The model under review builds one solid part; all positions refer to its coordinate system, in mm. Face numbers are marked on the shaded views. A direction names the side the tool comes from. Give positions to 0.01 mm unless a question says otherwise; leave off trailing zeros. Loops run counter-clockwise (first coordinate to the right, second up) from the corner with the lowest first, then second, coordinate; pieces in that order, holes last. Notation, with made-up numbers: (45, 74.5) - (89, 74.5) arc R11 ccw to (89, 82.5) - close; hole circle Ø6 at (45, 53.5). An arc over 180 degrees is marked (long way). Return JSON: item names as keys, results as strings. Group by question number.
```python
from build123d import *

# Parameters (mm, degrees)
EXTRUDE_1_DEPTH            = 48
CUT_EXTRUDE_2_REACH        = 96.508
CUT_EXTRUDE_2_START_RADIUS = 70
CUT_EXTRUDE_2_END_RADIUS   = 70
SKETCH_3_W                 = 58.404028666
SKETCH_3_H                 = 6
EXTRUDE_2_DEPTH            = 13
CUT_EXTRUDE_3_DEPTH        = 140.034418617
CUT_EXTRUDE_3_DEPTH_BACK   = 140.034418617
SKETCH_4_W                 = 25
SKETCH_4_H                 = 38
SKETCH_4_W_2               = 40
SKETCH_4_H_2               = 25
CHAMFER_1_SIZE             = 5
CHAMFER_1_SIZE2            = 3.813196151
SKETCH_6_R                 = 6.5
CUT_EXTRUDE_4_DEPTH        = 2
SKETCH_7_R                 = 1.5
CUT_EXTRUDE_5_DEPTH        = 60
SKETCH_8_W                 = 9
SKETCH_8_H                 = 9
CUT_EXTRUDE_6_DEPTH        = 11
CUT_EXTRUDE_8_REACH        = 137.533
SKETCH_10_R                = 1
CUT_EXTRUDE_9_REACH        = 105.034
CUT_EXTRUDE_9_END_RADIUS   = 70
SKETCH_11_R                = 0.75
SKETCH_12_W                = 20
SKETCH_12_H                = 3
CUT_EXTRUDE_10_DEPTH       = 11
SKETCH_13_W                = 3.868283576
SKETCH_13_H                = 1.5
CUT_EXTRUDE_11_DEPTH       = 4
CUT_EXTRUDE_12_REACH       = 137.476


with BuildPart() as part:
    # 草图1 → 凸台-拉伸1 (new body)
    with BuildSketch(Plane(origin=(0, 0, 0), x_dir=(1, 0, 0), z_dir=(0, 1, 0))):
        with BuildLine():
            ThreePointArc((-9.396926208, -7.075874358), (-5.735764364, -11.847193368), (0, -13.655672925))
            Line((0, -13.655672925), (0, -5))
            ThreePointArc((0, -5), (-5, 0), (0, 5))
            Line((0, 5), (0, 70))
            ThreePointArc((0, 70), (-17.673593853, 67.732149533), (-34.202014333, 61.075545152))
            Line((-34.202014333, 61.075545152), (-9.396926208, -7.075874358))
        make_face()
        with BuildLine():
            Line((0, -5), (0, -13.655672925))
            ThreePointArc((0, -13.655672925), (5.735764364, -11.847193368), (9.396926208, -7.075874358))
            Line((9.396926208, -7.075874358), (34.202014333, 61.075545152))
            ThreePointArc((34.202014333, 61.075545152), (17.673593853, 67.732149533), (0, 70))
            Line((0, 70), (0, 5))
            ThreePointArc((0, 5), (3.535533906, 3.535533906), (5, 0))
            ThreePointArc((5, 0), (3.535533906, -3.535533906), (0, -5))
        make_face()
    extrude(amount=EXTRUDE_1_DEPTH)

    # 切除-拉伸2: from a cylinder face, 96.508 long prism both ways, kept between that surface and its translate by the depth
    cut_extrude_2_start = Plane(origin=(0, 5, 0), z_dir=(0, -1, 0)) * Cylinder(CUT_EXTRUDE_2_START_RADIUS, 334.016, mode=Mode.PRIVATE)
    cut_extrude_2_end = Plane(origin=(0, 5, 3), z_dir=(0, -1, 0)) * Cylinder(CUT_EXTRUDE_2_END_RADIUS, 334.016, mode=Mode.PRIVATE)
    # 草图3 → 切除-拉伸2 (cut, from a surface)
    with BuildSketch(Plane.XY, mode=Mode.PRIVATE) as cut_extrude_2_sk1:
        with Locations((3, 5)):
            Rectangle(SKETCH_3_W, SKETCH_3_H)
    cut_extrude_2_tool1 = extrude(cut_extrude_2_sk1.sketch, amount=CUT_EXTRUDE_2_REACH, both=True, mode=Mode.PRIVATE)
    add(((cut_extrude_2_tool1 & cut_extrude_2_start) - cut_extrude_2_end).solids().sort_by_distance((3, 5, -62.032204))[0], mode=Mode.SUBTRACT)

    # 草图2 → 凸台-拉伸2 (add)
    with BuildSketch(Plane(origin=(0, 48, 0), x_dir=(1, 0, 0), z_dir=(0, 1, 0))):
        Polygon((24.252642572, 33.739870901), (55.034455471, 118.312206771), (20.125623779, 80.877067961), (5.458790156, 40.580273767), align=None)
    extrude(amount=-EXTRUDE_2_DEPTH)

    # 草图4 → 切除-拉伸3 (cut, two sides: drawn at the far end of the back side and taken through both)
    with BuildSketch(Plane(origin=(0, 0, 0), x_dir=(0, 0, -1), z_dir=(1, 0, 0)).offset(-CUT_EXTRUDE_3_DEPTH_BACK)):
        with Locations((-1.155672925, 29)):
            Rectangle(SKETCH_4_W, SKETCH_4_H)
        with Locations((50.466884927, 22.5)):
            Rectangle(SKETCH_4_W_2, SKETCH_4_H_2)
    extrude(amount=CUT_EXTRUDE_3_DEPTH + CUT_EXTRUDE_3_DEPTH_BACK, mode=Mode.SUBTRACT)

    # 倒角1
    chamfer_1_edges = [part.edges().sort_by_distance(p)[0] for p in [
        (55.034455471, 41.5, -118.312206771),
    ]]
    chamfer_1_side = [part.faces().sort_by_distance(p)[0] for p in [
        (37.580039625, 41.5, -99.594637366),
    ]]
    chamfer(chamfer_1_edges, length=CHAMFER_1_SIZE, length2=CHAMFER_1_SIZE2, reference=chamfer_1_side[0])

    # 草图6 → 切除-拉伸4 (cut)
    with BuildSketch(Plane.XZ):
        with Locations(Location((0, 0, 0), (0, 0, 270))):
            Circle(SKETCH_6_R)
    extrude(amount=-CUT_EXTRUDE_4_DEPTH, mode=Mode.SUBTRACT)

    # 草图7 → 切除-拉伸5 (cut)
    with BuildSketch(Plane.XY):
        with Locations((-30.202014333, 5)):
            Circle(SKETCH_7_R)
    extrude(amount=-CUT_EXTRUDE_5_DEPTH, mode=Mode.SUBTRACT)

    # 草图8 → 切除-拉伸6 (cut)
    with BuildSketch(Plane(origin=(0, 10, 0), x_dir=(1, 0, 0), z_dir=(0, 1, 0))):
        with Locations((-30.258231885, 50.240091929)):
            Rectangle(SKETCH_8_W, SKETCH_8_H)
    extrude(amount=-CUT_EXTRUDE_6_DEPTH, mode=Mode.SUBTRACT)

    # 切除-拉伸8: up to this plane
    cut_extrude_8_end = Plane(origin=(32.202014333, 48, -62.153280468), z_dir=(-1, 0, 0))
    # 草图10 → 切除-拉伸8 (cut, up to the surface)
    with BuildSketch(Plane(origin=(10.571836839, 0, 3.847833931), x_dir=(0.34202014332566283, 0, -0.9396926207859106), z_dir=(0.9396926207859106, 0, 0.34202014332566283)), mode=Mode.PRIVATE) as cut_extrude_8_sk1:
        with Locations((67.590016934, 5)):
            Circle(SKETCH_10_R)
    cut_extrude_8_tool1 = split(extrude(cut_extrude_8_sk1.sketch, amount=-CUT_EXTRUDE_8_REACH, mode=Mode.PRIVATE), bisect_by=cut_extrude_8_end, keep=Keep.BOTH, mode=Mode.PRIVATE)
    add(cut_extrude_8_tool1.solids().sort_by_distance((33.688984, 5, -59.666006))[0], mode=Mode.SUBTRACT)

    # 切除-拉伸9: up to this cylinder (the profile starts inside it)
    cut_extrude_9_end = Plane(origin=(0, 5, 0), z_dir=(0, -1, 0)) * Cylinder(CUT_EXTRUDE_9_END_RADIUS, 351.068, mode=Mode.PRIVATE)
    # 草图11 → 切除-拉伸9 (cut, up to the surface)
    with BuildSketch(Plane.XY.offset(-60), mode=Mode.PRIVATE) as cut_extrude_9_sk1:
        with Locations((-30.202014333, 5)):
            Circle(SKETCH_11_R)
    cut_extrude_9_tool1 = extrude(cut_extrude_9_sk1.sketch, amount=-CUT_EXTRUDE_9_REACH, mode=Mode.PRIVATE) & cut_extrude_9_end
    add(cut_extrude_9_tool1.solids().sort_by_distance((-30.202014, 5, -60))[0], mode=Mode.SUBTRACT)

    # 草图12 → 切除-拉伸10 (cut)
    with BuildSketch(Plane(origin=(0, 10, 0), x_dir=(1, 0, 0), z_dir=(0, 1, 0))):
        with Locations((8.346963974, 51.411545488)):
            Rectangle(SKETCH_12_W, SKETCH_12_H)
    extrude(amount=-CUT_EXTRUDE_10_DEPTH, mode=Mode.SUBTRACT)

    # 草图13 → 切除-拉伸11 (cut)
    with BuildSketch(Plane(origin=(0, 10, 0), x_dir=(1, 0, 0), z_dir=(0, 1, 0))):
        with Locations((29.542762739, 51.411545488)):
            Rectangle(SKETCH_13_W, SKETCH_13_H)
    extrude(amount=-CUT_EXTRUDE_11_DEPTH, mode=Mode.SUBTRACT)

    # 草图14 → 切除-拉伸12 (cut, up to next)
    with BuildSketch(Plane(origin=(0, 48, 0), x_dir=(1, 0, 0), z_dir=(0, 1, 0)), mode=Mode.PRIVATE) as cut_extrude_12_sk1:
        Polygon((49.766128767, 108.223290792), (49.034775066, 108.905289152), (40.168796385, 99.397691031), (40.900150086, 98.715692671), align=None)
    cut_extrude_12_tool1 = extrude(cut_extrude_12_sk1.sketch, amount=-CUT_EXTRUDE_12_REACH, mode=Mode.PRIVATE) & part.part
    add(cut_extrude_12_tool1.solids().sort_by_distance((44.967463, 48, -103.810491))[0], mode=Mode.SUBTRACT)


solid = part.part
```
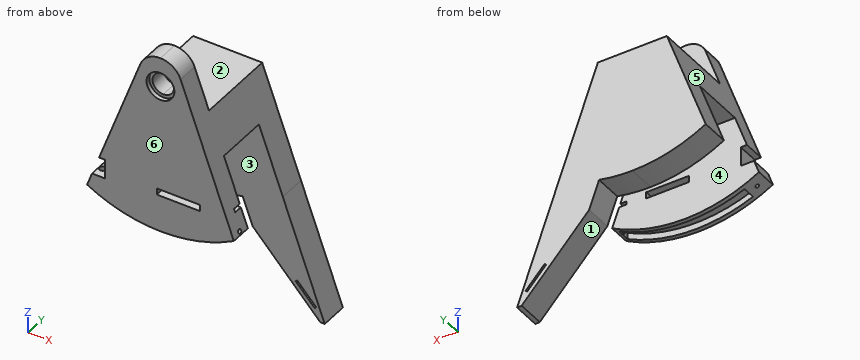
1) We need section D-D, the plane y = 20. Write out the cut boundary in (x, z), plus the area to 3 significant figures.
2) For pin 1 Ø4 at (x, y) = (-14.5, 42.5) entering from +Z; pin 2 Ø2.5 at (x, y) = (-28, 3.5) entering from -Z; pin 3 Ø1 at (y, z) = (7.5, -17.5) entering from -X, all flat-tipped, find the tip position at first contact; note any pin that passes through.
3) We need section C-C, the plane z = -37. Write out the cut boundary in (x, y), plus the area to 3 significant figures.
4) We need section B-B, the plane y = 45. Write out the cut boundary in (x, z), plus the area to 3 significant figures.
5) Draft analysis for pull direction Y (two halves, no side actions). For the marked faces 4, 5 and 6, state which applies: +Y half, -Y half, draft (parallel to the pull), parting line (faces both ways), or undercut.
6) To check wall thickness, follow line 1 (X direction, y = 5, z = -61.3); line 2 (Y direction, x = 28, z = -59); line 3 (Y direction, x = 28.5, z = -64.5). State the ranges of each line that lie inside material, in increasing order.
7) We need section A-A, the plane x = 47. Write out the cut boundary in (y, z).
8) Tool access review of the marked faces 1, 2 and 3: name each direction out of +Z, -Z, +X, -X, +Y, -Y from which nothing blocks a thin tool from reaching the whole face with its end or side.
Findings:
{
 "1": {"outline": "(-23.06, -30.47) - (23.06, -30.47) - (16.1, -11.34) - (-16.1, -11.34) - close", "area": "749 mm^2"},
 "2": {"pin 1": "stops at z = -11.34", "pin 2": "stops at z = -64.69", "pin 3": "stops at x = -18.52"},
 "3": {"outline": "(-25.44, 0) - (25.44, 0) - (25.44, 10) - (-25.44, 10) - close; (-25.44, 35) - (25.44, 35) - (25.44, 48) - (-25.44, 48) - close", "area": "1,170 mm^2"},
 "4": {"outline": "(-34.2, -61.08) arc R70 ccw to (15.53, -68.26) - (20.13, -80.88) - (51.62, -114.66) - (53.73, -114.73) - (16.1, -11.34) - (-16.1, -11.34) - close; hole (40.17, -99.4) - (49.03, -108.91) - (49.77, -108.22) - (40.9, -98.72) - close", "area": "3,630 mm^2"},
 "5": {"face 4": "undercut", "face 5": "draft", "face 6": "-Y half"},
 "6": {"line 1": "x = -33.8 to -30.95, -29.45 to 27.67, 32.2 to 33.8", "line 2": "y = 0 to 10, 35 to 48", "line 3": "y = 35 to 48"},
 "7": {"outline": "(35, -109.7) - (48, -109.7) - (48, -106.72) - (35, -106.72) - close; (35, -105.26) - (48, -105.26) - (48, -96.24) - (35, -96.24) - close"},
 "8": {"face 1": "-Z, -X, +Y, -Y", "face 2": "+Z, +X, -X, +Y", "face 3": "-Z, +X, -X"}
}
